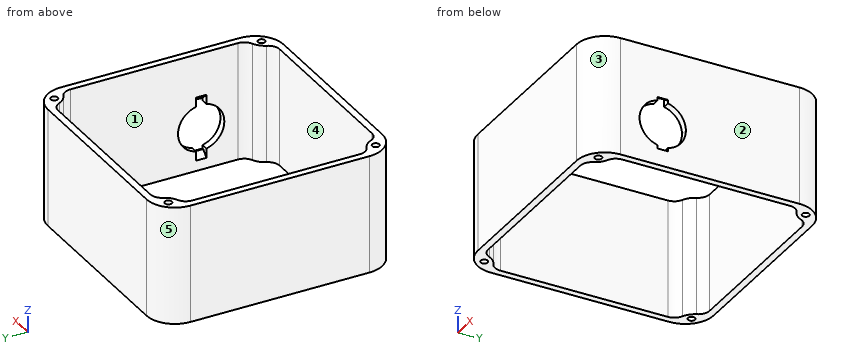
```python
from build123d import *

# Parameters (mm, degrees)
F0_R     = 1.5
F1_DEPTH = 50
F2_R     = 12
F3_R     = 5
F5_DEPTH = 4
F6_SIZE  = 2.5


with BuildPart() as f1:
    # F0 (on Top) → F1 (new body)
    with BuildSketch(Plane.XY):
        with BuildLine():
            Line((-50, 40.1261364576), (-50, -40.1261364576))
            ThreePointArc((-50, -40.1261364576), (-48.5323223277, -39.658202653), (-47, -39.5))
            Line((-47, -39.5), (-47, 39.5))
            ThreePointArc((-47, 39.5), (-48.5323223277, 39.658202653), (-50, 40.1261364576))
        make_face()
        with BuildLine():
            Line((-50, -50), (-40.1261364576, -50))
            ThreePointArc((-40.1261364576, -50), (-39.658202653, -48.5323223277), (-39.5, -47))
            Line((-39.5, -47), (-47, -47))
            Line((-47, -47), (-47, -39.5))
            ThreePointArc((-47, -39.5), (-48.5323223277, -39.658202653), (-50, -40.1261364576))
            Line((-50, -40.1261364576), (-50, -50))
        make_face()
        with BuildLine():
            Line((-47, -47), (-39.5, -47))
            ThreePointArc((-39.5, -47), (-41.6966991411, -41.6966991411), (-47, -39.5))
            Line((-47, -39.5), (-47, -47))
        make_face()
        with Locations((-44, -44)):
            Circle(F0_R, mode=Mode.SUBTRACT)
        with BuildLine():
            Line((-40.1261364576, -50), (40.1261364576, -50))
            ThreePointArc((40.1261364576, -50), (39.658202653, -48.5323223277), (39.5, -47))
            Line((39.5, -47), (-39.5, -47))
            ThreePointArc((-39.5, -47), (-39.658202653, -48.5323223277), (-40.1261364576, -50))
        make_face()
        with BuildLine():
            Line((40.1261364576, -50), (50, -50))
            Line((50, -50), (50, -40.1261364576))
            ThreePointArc((50, -40.1261364576), (48.5323223277, -39.658202653), (47, -39.5))
            Line((47, -39.5), (47, -47))
            Line((47, -47), (39.5, -47))
            ThreePointArc((39.5, -47), (39.658202653, -48.5323223277), (40.1261364576, -50))
        make_face()
        with BuildLine():
            ThreePointArc((47, -39.5), (41.6966991411, -41.6966991411), (39.5, -47))
            Line((39.5, -47), (47, -47))
            Line((47, -47), (47, -39.5))
        make_face()
        with Locations((44, -44)):
            Circle(F0_R, mode=Mode.SUBTRACT)
        with BuildLine():
            ThreePointArc((47, -39.5), (48.5323223277, -39.658202653), (50, -40.1261364576))
            Line((50, -40.1261364576), (50, 40.1261364576))
            ThreePointArc((50, 40.1261364576), (48.5323223277, 39.658202653), (47, 39.5))
            Line((47, 39.5), (47, -39.5))
        make_face()
        with BuildLine():
            ThreePointArc((47, 39.5), (48.5323223277, 39.658202653), (50, 40.1261364576))
            Line((50, 40.1261364576), (50, 50))
            Line((50, 50), (40.1261364576, 50))
            ThreePointArc((40.1261364576, 50), (39.658202653, 48.5323223277), (39.5, 47))
            Line((39.5, 47), (47, 47))
            Line((47, 47), (47, 39.5))
        make_face()
        with BuildLine():
            ThreePointArc((39.5, 47), (41.6966991411, 41.6966991411), (47, 39.5))
            Line((47, 39.5), (47, 47))
            Line((47, 47), (39.5, 47))
        make_face()
        with Locations((44, 44)):
            Circle(F0_R, mode=Mode.SUBTRACT)
        with BuildLine():
            ThreePointArc((39.5, 47), (39.658202653, 48.5323223277), (40.1261364576, 50))
            Line((40.1261364576, 50), (-40.1261364576, 50))
            ThreePointArc((-40.1261364576, 50), (-39.658202653, 48.5323223277), (-39.5, 47))
            Line((-39.5, 47), (39.5, 47))
        make_face()
        with BuildLine():
            Line((-50, 50), (-50, 40.1261364576))
            ThreePointArc((-50, 40.1261364576), (-48.5323223277, 39.658202653), (-47, 39.5))
            Line((-47, 39.5), (-47, 47))
            Line((-47, 47), (-39.5, 47))
            ThreePointArc((-39.5, 47), (-39.658202653, 48.5323223277), (-40.1261364576, 50))
            Line((-40.1261364576, 50), (-50, 50))
        make_face()
        with BuildLine():
            Line((-47, 47), (-47, 39.5))
            ThreePointArc((-47, 39.5), (-41.6966991411, 41.6966991411), (-39.5, 47))
            Line((-39.5, 47), (-47, 47))
        make_face()
        with Locations((-44, 44)):
            Circle(F0_R, mode=Mode.SUBTRACT)
    extrude(amount=F1_DEPTH)

    # F2
    f2_edges = [f1.edges().sort_by_distance(p)[0] for p in [
        (-50, 50, 25),
        (50, 50, 25),
        (50, -50, 25),
        (-50, -50, 25),
    ]]
    fillet(f2_edges, radius=F2_R)

    # F3
    f3_edges = [f1.edges().sort_by_distance(p)[0] for p in [
        (-47, -39.5, 25),
        (-39.5, -47, 25),
        (39.5, -47, 25),
        (47, -39.5, 25),
        (39.5, 47, 25),
        (47, 39.5, 25),
        (-47, 39.5, 25),
        (-39.5, 47, 25),
    ]]
    fillet(f3_edges, radius=F3_R)

    # F4 (on face) → F5 (cut)
    with BuildSketch(Plane.YZ.offset(50)):
        with BuildLine():
            Line((-22.25, 8.4361030432), (-22.25, 27.5638969568))
            ThreePointArc((-22.25, 27.5638969568), (-29.825, 18), (-22.25, 8.4361030432))
        make_face()
        with BuildLine():
            Line((-17.75, 8.4361030432), (-17.75, 27.5638969568))
            ThreePointArc((-17.75, 27.5638969568), (-20, 27.825), (-22.25, 27.5638969568))
            Line((-22.25, 27.5638969568), (-22.25, 8.4361030432))
            ThreePointArc((-22.25, 8.4361030432), (-20, 8.175), (-17.75, 8.4361030432))
        make_face()
        with BuildLine():
            ThreePointArc((-17.75, 8.4361030432), (-12.2981536305, 11.8998206994), (-10.175, 18))
            ThreePointArc((-10.175, 18), (-12.2981536305, 24.1001793006), (-17.75, 27.5638969568))
            Line((-17.75, 27.5638969568), (-17.75, 8.4361030432))
        make_face()
        with BuildLine():
            ThreePointArc((-22.25, 27.5638969568), (-20, 27.825), (-17.75, 27.5638969568))
            Line((-17.75, 27.5638969568), (-17.75, 29.05))
            Line((-17.75, 29.05), (-22.25, 29.05))
            Line((-22.25, 29.05), (-22.25, 27.5638969568))
        make_face()
        with BuildLine():
            Line((-17.75, 6.95), (-17.75, 8.4361030432))
            ThreePointArc((-17.75, 8.4361030432), (-20, 8.175), (-22.25, 8.4361030432))
            Line((-22.25, 8.4361030432), (-22.25, 6.95))
            Line((-22.25, 6.95), (-17.75, 6.95))
        make_face()
    extrude(amount=-F5_DEPTH, mode=Mode.SUBTRACT)

    # F6
    f6_edges = [f1.edges().sort_by_distance(p)[0] for p in [
        (47, -20, 29.05),
        (47, -20, 6.95),
    ]]
    chamfer(f6_edges, length=F6_SIZE)


solid = f1.part
```
Input: part model. Units: mm. Frame: model coordinates. Face numbers are marked on the shaded views. A direction names the side the tool comes from. Coordinates: 2 decimals unless noted, no trailing zeros. Loops run counter-clockwise (first coordinate to the right, second up) from the corner with the lowest first, then second, coordinate; pieces in that order, holes last. Notation, with made-up numbers: (71.25, -8) -> (118.25, -8) arc R24 ccw to (118.25, 27) -> close; hole circle Ø4 at (33, 10). An arc over 180 degrees is marked (long way). Use a Markdown table: item, result.
1) Contact query for flat-ended pins moving along their axis: pin 1 (1 mm diameter, centred on x = -40, z = 6, fed in from -Y); pin 2 (1.5 mm diameter, centred on x = 48.5, z = 30.5, fed in from +Y); pin 3 (3.5 mm diameter, centred on x = 49, z = 7.5, fed in from -Y); pin 4 (5 mm diameter, centred on x = 44, y = -44, fed in from -Z). Output: stop coordinate, or through.
Results found:
| item | result |
|---|---|
| pin 1 | stops at y = -49.91 |
| pin 2 | stops at y = 45 |
| pin 3 | stops at y = -45.64 |
| pin 4 | stops at z = 0 |
2) Access query for the marked faces 4 and 5. Directions: +Z, -Z, +X, -X, +Y, -Y. A direction counts if a zero-diameter tool reaches every point of the face in a straight line with its end or side. Return the directions, or none.
Results found:
| item | result |
|---|---|
| face 4 | +Z, -Z |
| face 5 | +Z, -Z, -X, +Y |
3) Cut plane C-C (z = 20). Give the number of separate pieces and of enclosed holes in the cut face, then the cut area to 3 significant figures.
Results found:
| item | result |
|---|---|
| separate pieces | 1 |
| enclosed holes | 4 |
| area | 1,150 mm2 |
4) Material intervals for line 1 along X through (y, z) = (30, 45); line 2 along Y through (x, z) = (44, 20.5), sorted ascending. Write a range as from..to.
Results found:
| item | result |
|---|---|
| line 1 | x = -50..-47, 47..50 |
| line 2 | y = -48.39..-45.5, -42.5..-40.13, 40.13..42.5, 45.5..48.39 |
5) Cut plane A-A (x = -33). Return the cut outline in (y, z).
Results found:
| item | result |
|---|---|
| outline | (-50, 0) -> (-47, 0) -> (-47, 50) -> (-50, 50) -> close; (47, 0) -> (50, 0) -> (50, 50) -> (47, 50) -> close |
6) Pull-direction query (Y, two-part tool) for the marked faces 1, 2 and 3; classes: released by +Y, released by -Y, zero draft, split by the parting line, or undercut.
Results found:
| item | result |
|---|---|
| face 1 | undercut |
| face 2 | zero draft |
| face 3 | released by -Y |
7) Cut plane B-B (z = 43). Return the cut outline in (x, y), then the cut area to 3 significant figures.
Results found:
| item | result |
|---|---|
| outline | (-50, -38) arc R12 ccw to (-38, -50) -> (38, -50) arc R12 ccw to (50, -38) -> (50, 38) arc R12 ccw to (38, 50) -> (-38, 50) arc R12 ccw to (-50, 38) -> close; hole (-47, -35.54) arc R5 ccw to (-44, -40.13) arc R7.5 cw to (-40.13, -44) arc R5 ccw to (-35.54, -47) -> (35.54, -47) arc R5 ccw to (40.13, -44) arc R7.5 cw to (44, -40.13) arc R5 ccw to (47, -35.54) -> (47, 35.54) arc R5 ccw to (44, 40.13) arc R7.5 cw to (40.13, 44) arc R5 ccw to (35.54, 47) -> (-35.54, 47) arc R5 ccw to (-40.13, 44) arc R7.5 cw to (-44, 40.13) arc R5 ccw to (-47, 35.54) -> close; hole circle Ø3 at (-44, -44); hole circle Ø3 at (-44, 44); hole circle Ø3 at (44, -44); hole circle Ø3 at (44, 44) |
| area | 1,210 mm2 |
